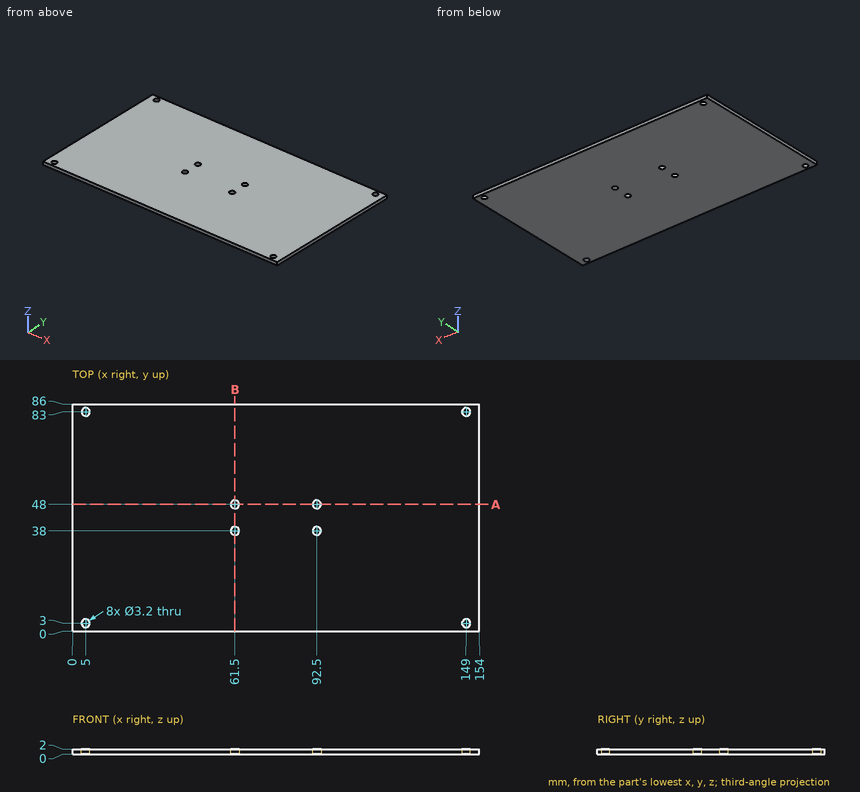
Verification items for this drawing (mm, ordinates from the low corner). Give positions to 0.01 mm unless a question says otherwise; leave off trailing zeros. Loops run counter-clockwise (first coordinate to the right, second up) from the corner with the lowest first, then second, coordinate; pieces in that order, holes last. Notation, with made-up numbers: M 49,-11 L 65,-11 A18 ccw 65,6 Z; hole C 59,12.25 d9. An arc over 180 degrees is marked long. Write item = value, one per line.
(1) Sectioned sample at A-A, the plane y = 48. Record the cut outline in (x, z).
Answer below:
outline = M 0,0 L 59.9,0 L 59.9,2 L 0,2 Z; M 63.1,0 L 90.9,0 L 90.9,2 L 63.1,2 Z; M 94.1,0 L 154,0 L 154,2 L 94.1,2 Z
(2) Gauge pin test, flat end, axial feed: pin 1 Ø4 at (x, y) = (5, 3) entering from -Z. Record the tip position at first contact, or that the pin passes through.
Answer below:
pin_1 = 0
(3) Sectioned sample at B-B, the plane x = 61.5. Record the cut outline in (y, z).
Answer below:
outline = M 0,0 L 36.4,0 L 36.4,2 L 0,2 Z; M 39.6,0 L 46.4,0 L 46.4,2 L 39.6,2 Z; M 49.6,0 L 86,0 L 86,2 L 49.6,2 Z
(4) Material ranges on line 1 (Y direction, x = 5, z = 0.5); line 2 (Y direction, x = 61.5, z = 1.3); line 3 (X direction, y = 47, z = 1.3), recorded low to high. Write a range as [from, to].
Answer below:
line_1 = [0, 1.4], [4.6, 81.4], [84.6, 86]
line_2 = [0, 36.4], [39.6, 46.4], [49.6, 86]
line_3 = [0, 60.25], [62.75, 91.25], [93.75, 154]
